```python
from build123d import *

# Parameters (mm, degrees)
BOSS_EXTRUDE1_DEPTH = 30
SKETCH2_R           = 25
CUT_EXTRUDE1_DEPTH  = 30
SKETCH3_R           = 6.505
BOSS_EXTRUDE2_DEPTH = 40


with BuildPart() as part:
    # Sketch1 → Boss-Extrude1 (new body)
    with BuildSketch(Plane(origin=(0, 0, 0), x_dir=(1, 0, 0), z_dir=(0, 1, 0))):
        with BuildLine():
            Line((-77.61802258, 0), (-33.820586084, 266.179413916))
            ThreePointArc((-33.820586084, 266.179413916), (0, 300), (33.820586084, 266.179413916))
            Line((33.820586084, 266.179413916), (72.176610565, 0))
            Line((72.176610565, 0), (33.820586084, -266.179413916))
            ThreePointArc((33.820586084, -266.179413916), (0, -300), (-33.820586084, -266.179413916))
            Line((-33.820586084, -266.179413916), (-77.61802258, 0))
        make_face()
    extrude(amount=BOSS_EXTRUDE1_DEPTH)

    # Sketch2 → Cut-Extrude1 (cut)
    with BuildSketch(Plane(origin=(0, 30, 0), x_dir=(1, 0, 0), z_dir=(0, 1, 0))):
        Circle(SKETCH2_R)
    extrude(amount=-CUT_EXTRUDE1_DEPTH, mode=Mode.SUBTRACT)

    # Sketch3 → Boss-Extrude2 (add)
    with BuildSketch(Plane(origin=(0, 30, 0), x_dir=(1, 0, 0), z_dir=(0, 1, 0))):
        with Locations((0, -280)):
            Circle(SKETCH3_R)
    extrude(amount=BOSS_EXTRUDE2_DEPTH)


solid = part.part
```
Geometry check sheet. Reference: the model listing, model coordinates, mm. A direction names the side the tool comes from. Coordinates: 2 decimals unless noted, no trailing zeros. Order: outer loops, then holes, each group sorted by start corner. A loop starts at its lowest first (then second) coordinate and runs counter-clockwise, first axis right, second up. Notation, with made-up numbers: (5.25, 10) - (18.25, 10) arc R29 cw to (18.25, 41) - close; hole circle Ø11 at (39.5, -6.75). An arc over 180 degrees is marked (long way). Answer as a JSON object with one key per item and string values. Group by question number.
Item 1: Sectioned sample at C-C, the plane z = 280. Record the cut outline in (x, y) (3 decimals), and give its area (3 significant figures).
Item 2: Draft check along X on faces 3 (the face through (23.846, 15.21, -7.509)), 4 (the face through (32, 30, -4)), 5 (the face through (0.74, 14.79, 299.99)), 6 (the face through (-55.413, 14.79, 134.953)). Enter one of: +X half, -X half, draft (parallel to the pull), parting line (faces both ways), or undercut.
Item 3: Tool access check on faces 1 (the face through (-56.026, 14.79, -131.226)), 2 (the face through (-0.85, 49.72, 273.55)). Record the directions out of +Z, -Z, +X, -X, +Y, -Y that give a thin tool (end or side, any length) a straight path to the whole face; none if there is none.
Item 4: Sectioned sample at A-A, the plane x = 0. Record the cut outline in (y, z) (3 decimals).
Item 5: Depth check by flat-ended pin: pin 1 Ø10 at (x, z) = (41.5, -10) entering from +Y; pin 2 Ø1 at (x, y) = (24.5, 26) entering from -Z; pin 3 Ø10 at (y, z) = (26.5, -106.5) entering from +X; pin 4 Ø1 at (x, z) = (-14, -97) entering from -Y. Enter the tip coordinate at first touch or a pass-through.
Item 6: Sectioned sample at B-B, the plane y = 12. Record the cut outline in (x, z), and give its area (3 significant figures).
Item 7: Scan lines: probe 1 along X at (y, z) = (14, 0); probe 2 along Z at (x, y) = (0, 22); probe 3 along Y at (x, z) = (-17, 57). Record each from-to range of solid material in increasing order.
Item 8: Sectioned sample at D-D, the plane y = 40.5. Record the cut outline in (x, z) (3 decimals), and give its area (3 significant figures).
Resolved:
{
 "1": {"outline": "(-30.868, 0) - (30.868, 0) - (30.868, 30) - (6.505, 30) - (6.505, 70) - (-6.505, 70) - (-6.505, 30) - (-30.868, 30) - close", "area": "2,370 mm^2"},
 "2": {"face 3": "undercut", "face 4": "draft", "face 5": "parting line", "face 6": "-X half"},
 "3": {"face 1": "-Z, -X, +Y, -Y", "face 2": "+Y"},
 "4": {"outline": "(0, -300) - (30, -300) - (30, -25) - (0, -25) - close; (0, 25) - (30, 25) - (30, 273.495) - (70, 273.495) - (70, 286.505) - (30, 286.505) - (30, 300) - (0, 300) - close"},
 "5": {"pin 1": "y = 30", "pin 2": "z = -290.01", "pin 3": "x = 57.55", "pin 4": "y = 0"},
 "6": {"outline": "(-77.62, 0) - (-33.82, -266.18) arc R33.82 ccw to (33.82, -266.18) - (72.18, 0) - (33.82, 266.18) arc R33.82 ccw to (-33.82, 266.18) - close; hole circle Ø50 at (0, 0)", "area": "59,500 mm^2"},
 "7": {"probe 1": "-77.62 to -25, 25 to 72.18", "probe 2": "-300 to -25, 25 to 300", "probe 3": "0 to 30"},
 "8": {"outline": "circle Ø13.01 at (0, 280)", "area": "133 mm^2"}
}
